Design review of the part built by this model. Coordinates are the model's own, in mm. A direction names the side the tool comes from. Coordinates: 2 decimals unless noted, no trailing zeros. Loops run counter-clockwise (first coordinate to the right, second up) from the corner with the lowest first, then second, coordinate; pieces in that order, holes last.
from build123d import *

# Parameters (mm, degrees)
F1_DEPTH = 20
F2_R     = 4
F3_DEPTH = 5


with BuildPart() as f1:
    # F0 (on Front) → F1 (new body)
    with BuildSketch(Plane.XZ):
        Polygon((0, 40), (0, 0), (60, 0), align=None)
    extrude(amount=F1_DEPTH)

    # F2 (on face) → F3 (cut)
    with BuildSketch(Plane(origin=(0, 0, 0), x_dir=(0, -1, 0), z_dir=(-1, 0, 0))):
        with Locations((10, 7)):
            Circle(F2_R)
        with Locations((10, 27)):
            Circle(F2_R)
    extrude(amount=-F3_DEPTH, mode=Mode.SUBTRACT)


solid = f1.part
Q1. Take a section at B-B, the plane y = -10. Write out the cut boundary in (x, z).
Q2. For line 1 (Z direction, x = 3.8, y = -10); line 2 (Z direction, x = 3.95, y = -10); line 3 (Z direction, x = 55.5, y = -4.5), list the stretches that pass through material, from the lowest coordinate up.
Q3. Clearance check with flat-ended pins moving along their axes: pin 1 Ø10 at (x, y) = (14.5, -14.5) entering from +Z; pin 2 Ø9 at (y, z) = (-10, 7) entering from +X; pin 3 Ø3 at (y, z) = (-12.5, 5) entering from +X. State where each tip first meets the part, or that it passes through.
Q4. Take a section at A-A, the plane z = 27. Write out the cut boundary in (x, y).
Q5. Machinability: for faces 1 (the flat face through (0, -10, 20)), 2 (the flat face through (5, -10, 7)), which of the approach directions +Z, -Z, +X, -X, +Y, -Y give a long, thin tool a straight path to every point of the face, cutting with its end or side? Answer none if there is none.
Q6. Take a section at C-C, the plane x = 40.5. Write out the cut boundary in (y, z).
Q7. Take a section at D-D, the plane z = 7. Write out the cut boundary in (x, y), then the cut area to 3 significant figures.
Q8. The part is to be moulded in two halves that separate along Y. For faces 3 (the flat face through (5, -10, 27)), 4 (the flat face through (30, -10, 20)), 5 (the flat face through (16, -20, 11)), 6 (the flat face through (16, 0, 11)), say which applies: pulls with the +Y half, pulls with the -Y half, needs draft (parallel to the pull), parting line crosses it, or undercut.
Entries:
1. outline: (0, 0) - (60, 0) - (0, 40) - (0, 31) - (5, 31) - (5, 23) - (0, 23) - (0, 11) - (5, 11) - (5, 3) - (0, 3) - close
2. line 1: z = 0 to 3, 11 to 23, 31 to 37.47
2. line 2: z = 0 to 3, 11 to 23, 31 to 37.37
2. line 3: z = 0 to 3
3. pin 1: stops at z = 33.67
3. pin 2: stops at x = 56.25
3. pin 3: stops at x = 54.75
4. outline: (0, -20) - (19.5, -20) - (19.5, 0) - (0, 0) - (0, -6) - (5, -6) - (5, -14) - (0, -14) - close
5. face 1: +Z, -Z, -X, +Y, -Y
5. face 2: -X
6. outline: (-20, 0) - (0, 0) - (0, 13) - (-20, 13) - close
7. outline: (0, -20) - (49.5, -20) - (49.5, 0) - (0, 0) - (0, -6) - (5, -6) - (5, -14) - (0, -14) - close
7. area: 950 mm2
8. face 3: undercut
8. face 4: needs draft
8. face 5: pulls with the -Y half
8. face 6: pulls with the +Y half
